from build123d import *

# Parameters (mm, degrees)
F0_R     = 0.5
F1_DEPTH = 6


with BuildPart() as f1:
    # F0 (on Top) → F1 (new body)
    with BuildSketch(Plane.XY):
        with BuildLine():
            Line((18, 30.9), (-18, 30.9))
            ThreePointArc((-18, 30.9), (-20.828427, 29.728427), (-22, 26.9))
            Line((-22, 26.9), (-22, -26.9))
            ThreePointArc((-22, -26.9), (-20.828427, -29.728427), (-18, -30.9))
            Line((-18, -30.9), (18, -30.9))
            ThreePointArc((18, -30.9), (20.828427, -29.728427), (22, -26.9))
            Line((22, -26.9), (22, 26.9))
            ThreePointArc((22, 26.9), (20.828427, 29.728427), (18, 30.9))
        make_face()
        with Locations((-5, -24.375)):
            Circle(F0_R, mode=Mode.SUBTRACT)
        with Locations((5, -24.375)):
            Circle(F0_R, mode=Mode.SUBTRACT)
        with Locations((-5, 24.375)):
            Circle(F0_R, mode=Mode.SUBTRACT)
        Polygon((-16.5, 20.9), (-10.5, 20.9), (10.5, 20.9), (16.5, 20.9), (16.5, 15.1), (10.5, 15.1), (10.5, 8.9), (16.5, 8.9), (16.5, 3.1), (10.5, 3.1), (10.5, -3.1), (16.5, -3.1), (16.5, -8.9), (10.5, -8.9), (10.5, -15.1), (16.5, -15.1), (16.5, -20.9), (10.5, -20.9), (-10.5, -20.9), (-16.5, -20.9), (-16.5, -15.1), (-10.5, -15.1), (-10.5, -8.9), (-16.5, -8.9), (-16.5, -3.1), (-10.5, -3.1), (-10.5, 3.1), (-16.5, 3.1), (-16.5, 8.9), (-10.5, 8.9), (-10.5, 15.1), (-16.5, 15.1), align=None, mode=Mode.SUBTRACT)
        with Locations((5, 24.375)):
            Circle(F0_R, mode=Mode.SUBTRACT)
    extrude(amount=F1_DEPTH)


solid = f1.part
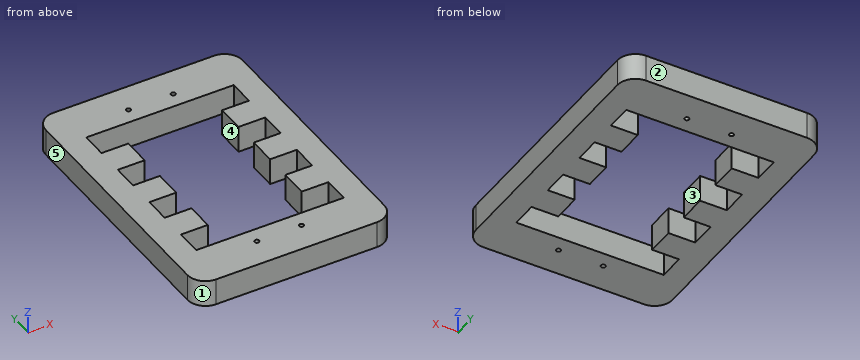
Geometry check sheet. Reference: the model listing, model coordinates, mm. Face numbers are marked on the shaded views. A direction names the side the tool comes from. Give positions to 0.01 mm unless a question says otherwise; leave off trailing zeros. Loops run counter-clockwise (first coordinate to the right, second up) from the corner with the lowest first, then second, coordinate; pieces in that order, holes last. Notation, with made-up numbers: (-33, 62.25) -> (9, 62.25) arc R21 ccw to (9, 95.25) -> close; hole circle Ø9 at (-37, -26). An arc over 180 degrees is marked (long way). Answer in a Markdown table with one row per item. Add a question column.
1) Cross-section at A-A on y = -8. Record the boundary of the cut face in (x, z).
2) Set-up check for the marked faces 4 and 5: record each of +Z, -Z, +X, -X, +Y, -Y from which the full face is reachable in a straight line by a thin tool's end or side.
3) Cross-section at D-D on z = 4.2. State how many separate pieces and enclosed holes the cut face has, and give its area (3 significant figures).
4) Material ranges on probe 1 along Y at (x, z) = (5, 4.1) (3 decimals); probe 2 along Y at (x, z) = (12.5, 5.45); probe 3 along Y at (x, z) = (4, 2.95), recorded low to high. Write a range as from..to.
5) Cross-section at B-B on x = 8. Record the boundary of the cut face in (y, z).
6) Cross-section at C-C on x = -15. Record the boundary of the cut face in (y, z).
7) Draft check along Y on the marked faces 1, 2 and 3. Enter one of: pulls with the +Y half, pulls with the -Y half, needs draft (parallel to the pull), parting line crosses it, or undercut.
Outcome:
| question | item | result |
|---|---|---|
| 1 | outline | (-22, 0) -> (-16.5, 0) -> (-16.5, 6) -> (-22, 6) -> close; (16.5, 0) -> (22, 0) -> (22, 6) -> (16.5, 6) -> close |
| 2 | face 4 | +Z, -Z |
| 2 | face 5 | +Z, -Z, -X, +Y, -Y |
| 3 | separate pieces | 1 |
| 3 | enclosed holes | 5 |
| 3 | area | 1,550 mm^2 |
| 4 | probe 1 | y = -30.9..-24.875, -23.875..-20.9, 20.9..23.875, 24.875..30.9 |
| 4 | probe 2 | y = -30.9..-20.9, -15.1..-8.9, -3.1..3.1, 8.9..15.1, 20.9..30.9 |
| 4 | probe 3 | y = -30.9..-20.9, 20.9..30.9 |
| 5 | outline | (-30.9, 0) -> (-20.9, 0) -> (-20.9, 6) -> (-30.9, 6) -> close; (20.9, 0) -> (30.9, 0) -> (30.9, 6) -> (20.9, 6) -> close |
| 6 | outline | (-30.9, 0) -> (-20.9, 0) -> (-20.9, 6) -> (-30.9, 6) -> close; (-15.1, 0) -> (-8.9, 0) -> (-8.9, 6) -> (-15.1, 6) -> close; (-3.1, 0) -> (3.1, 0) -> (3.1, 6) -> (-3.1, 6) -> close; (8.9, 0) -> (15.1, 0) -> (15.1, 6) -> (8.9, 6) -> close; (20.9, 0) -> (30.9, 0) -> (30.9, 6) -> (20.9, 6) -> close |
| 7 | face 1 | pulls with the -Y half |
| 7 | face 2 | pulls with the +Y half |
| 7 | face 3 | undercut |
